Autodesk Inventor part; units mm, degrees
ref_plane "YZ Plane" through (0, 0, 0) normal (1, 0, 0) x (0, 1, 0)
ref_plane "XZ Plane" through (0, 0, 0) normal (0, 1, 0) x (-1, 0, 0)
ref_plane "XY Plane" through (0, 0, 0) normal (0, 0, 1) x (1, 0, 0)
sketch "スケッチ1" plane through (0, 0, 0) normal (0, 1, 0) x (-1, 0, 0)
  circle A0 centre (0, 0) radius 3
  dimension "d0" = 6
extrude "押し出し1" add sketch "スケッチ1" along normal mid plane 12
sketch "スケッチ2" plane through (0, 6, 0) normal (0, 1, 0) x (1, 0, 0)
  point P0 (0, 0)
  point P1 (0, 0)
hole "穴1" at (0, 6, 0) direction (0, -1, 0) diameter 2.459 depth 10 countersink diameter 3.4 countersink angle 90
sketch "スケッチ3" plane through (0, -6, 0) normal (0, -1, 0) x (1, 0, 0)
  point P0 (0, 0)
  point P1 (0, 0)
hole "穴2" at (0, -6, 0) direction (0, 1, 0) diameter 2.459 depth 10 countersink diameter 3.4 countersink angle 90
chamfer "面取り1" distance 0.25 angle 45 2 edges at (3, -6, 0) (3, 6, 0)
properties part number "Spacer_M3D6L60" material "アルミニウム 6061"
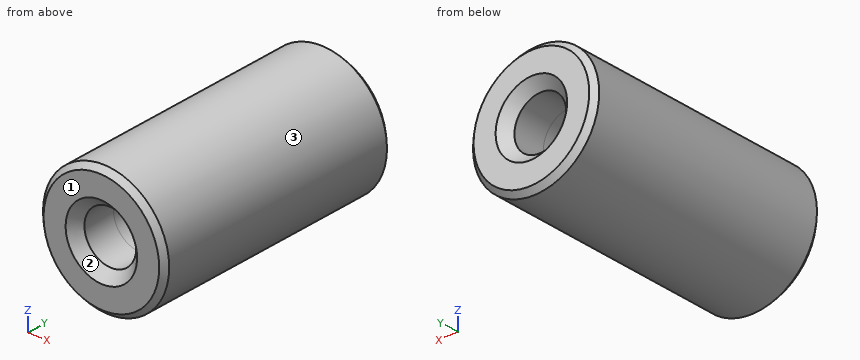
For this review, take the finished solid that the model builds, in its own axes (mm). Face numbers are marked on the shaded views. Give positions to 0.01 mm unless a question says otherwise; leave off trailing zeros. Write each loop counter-clockwise with the first axis right and the second up, starting at its lowest first coordinate (ties: lowest second). Pieces come first, ordered by that corner, then holes.
Item 1: The part is to be moulded in two halves that separate along X. For the marked faces 1, 2 and 3, say which applies: +X half, -X half, draft (parallel to the pull), parting line (faces both ways), or undercut.
Item 2: Insertion check: P1, Ø2, axis at x = 1.5, y = 0.5, coming from the +Z side; P2, Ø3, axis at x = 0, z = 0, coming from the +Y side; P3, Ø3, axis at x = 0, z = 0, coming from the -Y side. Each pin has a flat end and moves straight along its axis. Give the tip position at first contact, or say it passes through.
Item 3: Wall thickness on probe 1 along Z at (x, y) = (0, 4.3); probe 2 along Z at (x, y) = (-0.8, 1.75); probe 3 along X at (y, z) = (-2.75, -0.4): over which ranges is each line inside the solid? List them lowest first.
Item 4: Take a section at B-B (y = -1.5). Give the boundary of the cut face in (x, z), and give its area (3 significant figures).
Item 5: Take a section at A-A (z = 0). Give the boundary of the cut face in (x, y).
Established:
1. face 1: draft
1. face 2: undercut
1. face 3: parting line
2. P1: stops at z = 2.96
2. P2: stops at y = 5.8
2. P3: stops at y = -5.8
3. probe 1: z = -3 to -1.23, 1.23 to 3
3. probe 2: z = -2.89 to -0.93, 0.93 to 2.89
3. probe 3: x = -2.97 to -1.16, 1.16 to 2.97
4. outline: circle Ø6 at (0, 0); hole circle Ø2.46 at (0, 0)
4. area: 23.5 mm2
5. outline: (-3, -5.75) - (-2.75, -6) - (-1.7, -6) - (-1.23, -5.53) - (-1.23, 5.53) - (-1.7, 6) - (-2.75, 6) - (-3, 5.75) - close; (1.23, -5.53) - (1.7, -6) - (2.75, -6) - (3, -5.75) - (3, 5.75) - (2.75, 6) - (1.7, 6) - (1.23, 5.53) - close
